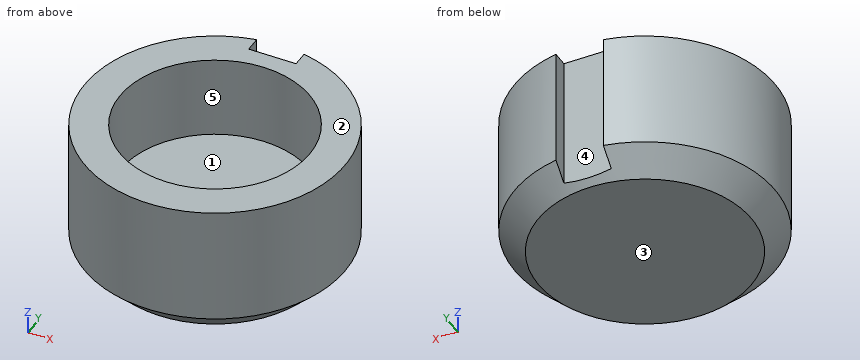
```python
from build123d import *

# Parameters (mm, degrees)
SKETCH1_R           = 11
BOSS_EXTRUDE1_DEPTH = 12
SKETCH2_R           = 8
CUT_EXTRUDE1_DEPTH  = 7
CHAMFER1_SIZE       = 2
SKETCH3_W           = 4
SKETCH3_H           = 3.288893808
CUT_EXTRUDE2_DEPTH  = 22


with BuildPart() as part:
    # Sketch1 → Boss-Extrude1 (new body)
    with BuildSketch(Plane.XY):
        Circle(SKETCH1_R)
    extrude(amount=BOSS_EXTRUDE1_DEPTH)

    # Sketch2 → Cut-Extrude1 (cut)
    with BuildSketch(Plane.XY.offset(12)):
        Circle(SKETCH2_R)
    extrude(amount=-CUT_EXTRUDE1_DEPTH, mode=Mode.SUBTRACT)

    # Chamfer1
    chamfer1_edges = [part.edges().sort_by_distance(p)[0] for p in [
        (-11, 0, 0),
    ]]
    chamfer(chamfer1_edges, length=CHAMFER1_SIZE)

    # Sketch3 → Cut-Extrude2 (cut)
    with BuildSketch(Plane.XY.offset(12)):
        with Locations((0, 11.144446904)):
            Rectangle(SKETCH3_W, SKETCH3_H)
    extrude(amount=-CUT_EXTRUDE2_DEPTH, mode=Mode.SUBTRACT)


solid = part.part
```
CAD build for the part. Positions are in the model's coordinates, mm. Face numbers are marked on the shaded views. A direction names the side the tool comes from. Round coordinates to 2 decimals unless told otherwise and drop trailing zeros. Loops run counter-clockwise (first coordinate to the right, second up) from the corner with the lowest first, then second, coordinate; pieces in that order, holes last. Notation, with made-up numbers: M 25.25,63.25 L 72.25,63.25 A12 ccw 72.25,69.25 Z; hole C 74.5,70 d4. An arc over 180 degrees is marked long. Return JSON: item names as keys, results as strings. Group by question number.
(1) Saw through at B-B, the plane z = 10.5. List the corners of the cut face in (x, y).
(2) Drop flat-ended pins along their axis: P1, Ø0.7, axis at y = 10, z = 7, coming from the +X side; P2, Ø5, axis at y = -4, z = 2.5, coming from the +X side; P3, Ø6, axis at x = 8.5, z = 10.5, coming from the -Y side. Give the stop position or say it passes through.
(3) Saw through at A-A, the plane y = 0. List the corners of the cut face in (x, z).
(4) Wall check: probe 1 along Y at (x, z) = (0, 9.25); probe 2 along Z at (x, y) = (4.25, 3.75); probe 3 along Y at (x, z) = (-2.5, 10). Give the ranges that are in metal, low to high. Write a range as [from, to].
(5) Tool access for the marked faces 1 and 2: list every direction of +Z, -Z, +X, -X, +Y, -Y with a clear straight run to the whole face (end or side of a thin tool).
(6) Saw through at C-C, the plane x = 0. List the corners of the cut face in (y, z), and give its area (3 significant figures).
(7) Mould opens along Y. For the marked faces 3, 4 and 5 say: +Y half, -Y half, draft (parallel to the pull), parting line (faces both ways), or undercut.
Answer list:
{
 "1": {"outline": "M -2,9.5 L -2,10.82 A11 ccw long 2,10.82 L 2,9.5 Z; hole C 0,0 d16"},
 "2": {"P1": "x = 5.28", "P2": "x = 10.9", "P3": "y = -9.53"},
 "3": {"outline": "M -11,2 L -9,0 L 9,0 L 11,2 L 11,12 L 8,12 L 8,5 L -8,5 L -8,12 L -11,12 Z"},
 "4": {"probe 1": "[-11, -8], [8, 9.5]", "probe 2": "[0, 5]", "probe 3": "[-10.71, -7.6], [7.6, 10.71]"},
 "5": {"face 1": "+Z", "face 2": "+Z, +X, -X, +Y, -Y"},
 "6": {"outline": "M -11,2 L -9,0 L 9,0 L 9.5,0.5 L 9.5,12 L 8,12 L 8,5 L -8,5 L -8,12 L -11,12 Z", "area": "132 mm2"},
 "7": {"face 3": "draft", "face 4": "+Y half", "face 5": "undercut"}
}
